Could you check a few things on this model? Use its own coordinates, in mm. A direction names the side the tool comes from. Give positions to 0.01 mm unless a question says otherwise; leave off trailing zeros. Order: outer loops, then holes, each group sorted by start corner. A loop starts at its lowest first (then second) coordinate and runs counter-clockwise, first axis right, second up. Notation, with made-up numbers: (-4.5, 7.5) - (28.5, 7.5) arc R22 cw to (28.5, 33.5) - close; hole circle Ø9 at (-11, -29). An arc over 180 degrees is marked (long way). Put each result on its own line as item: value.
from build123d import *

# Parameters (mm, degrees)
F0_R     = 3
F1_DEPTH = 50
F0_R_2   = 5
F2_DEPTH = 6
F4_DEPTH = 4
F5_R     = 0.2
F6_R     = 1


with BuildPart() as f1:
    # F0 (on Front) → F1 (new body)
    with BuildSketch(Plane.XZ):
        Circle(F0_R)
    extrude(amount=F1_DEPTH)

    # F0 (on Front) → F2 (join)
    with BuildSketch(Plane.XZ):
        Circle(F0_R_2)
        Circle(F0_R, mode=Mode.SUBTRACT)
        Circle(F0_R)
    extrude(amount=-F2_DEPTH)

    # F3 (on face) → F4 (cut)
    with BuildSketch(Plane(origin=(0, 6, 0), x_dir=(-1, 0, 0), z_dir=(0, 1, 0))):
        Polygon((2.196781, 1.872829), (-0.523527, 2.838882), (-2.720308, 0.966054), (-2.196781, -1.872829), (0.523527, -2.838882), (2.720308, -0.966054), align=None)
    extrude(amount=-F4_DEPTH, mode=Mode.SUBTRACT)

    # F5
    f5_edges = [f1.edges().sort_by_distance(p)[0] for p in [
        (-5, 6, 0),
        (-5, 0, 0),
        (0.836627, 6, -2.355855),
        (-1.621917, 6, -1.902468),
        (-2.458544, 6, 0.453387),
        (2.458544, 6, -0.453387),
        (1.621917, 6, 1.902468),
        (-0.836627, 6, 2.355855),
        (-1.621917, 2, -1.902468),
        (0.836627, 2, -2.355855),
        (2.458544, 2, -0.453387),
        (0.523527, 4, 2.838882),
        (2.720308, 4, 0.966054),
        (1.621917, 2, 1.902468),
        (-0.836627, 2, 2.355855),
        (-2.458544, 2, 0.453387),
    ]]
    fillet(f5_edges, radius=F5_R)

    # F6
    f6_edges = [f1.edges().sort_by_distance(p)[0] for p in [
        (-3, -50, 0),
    ]]
    fillet(f6_edges, radius=F6_R)


solid = f1.part
1) Which directions (+Z, -Z, +X, -X, +Y, -Y) give clear straight access to the entire face, cutting with the end or side of a thin tool? Please do faces 4 (the flat face through (0, -50, 0)), 5 (the cylindrical face through (0.8, 2.06, -2.31)), 6 (the flat face through (1, 0, -3)).
Filled in:
face 4: +Z, -Z, +X, -X, -Y
face 5: +Y
face 6: -Y
2) We'd pull the mould along Z, two halves only. Please class faces 1 (the cylindrical face through (-3, -24, 0)), 2 (the flat face through (-2.2, 6, -2.1)), 3 (the cylindrical face through (1.675, 5.943, 1.936)): pulls with the +Z half, pulls with the -Z half, needs draft (parallel to the pull), parting line crosses it, or undercut.
Filled in:
face 1: parting line crosses it
face 2: needs draft
face 3: undercut
3) Suppose I cut it at A-A, the plane y = 1. List the corners of the cut face in (x, z) for me.
Filled in:
outline: circle Ø10 at (0, 0)
4) Suppose I cut it at B-B, the plane y = -43.5. List the corners of the cut face in (x, z) for me.
Filled in:
outline: circle Ø6 at (0, 0)
5) I'm going to push flat-ended pins straight in: pin 1 (1 mm diameter, centred on x = 2.5, y = -7.5, fed in from -Z); pin 2 (4 mm diameter, centred on y = -6, z = 0, fed in from +X); pin 3 (3 mm diameter, centred on y = -42, z = -1.5, fed in from -X). Where does each tip first touch, or does it pass through?
Filled in:
pin 1: stops at z = -2.24
pin 2: stops at x = 3
pin 3: stops at x = -3
6) If I drill on line 1 (Y direction, x = 2.5, z = 3); line 2 (X direction, y = -17.5, z = -0.25), over which ranges is the centre line in solid material (lowest first)? Write a range as [from, to].
Filled in:
line 1: y = [0, 6]
line 2: x = [-2.99, 2.99]
